from build123d import *

# Parameters (mm, degrees)
SKETCH1_R           = 2
BOSS_EXTRUDE1_DEPTH = 3.5
BOSS_EXTRUDE3_START = -1
BOSS_EXTRUDE3_DEPTH = 2
FILLET1_R           = 1


with BuildPart() as part:
    # Sketch1 → Boss-Extrude1 (new body)
    with BuildSketch(Plane.XY):
        with BuildLine():
            Line((-63.221147144, 4.5), (-2.221147144, 4.5))
            ThreePointArc((-2.221147144, 4.5), (1.924633844, -3.295084972), (-6.856271198, -2.375))
            ThreePointArc((-6.856271198, -2.375), (-7.960294648, -1.012531407), (-9.637345631, -0.5))
            Line((-9.637345631, -0.5), (-55.804948657, -0.5))
            ThreePointArc((-55.804948657, -0.5), (-57.48199964, -1.012531407), (-58.586023089, -2.375))
            ThreePointArc((-58.586023089, -2.375), (-67.366928132, -3.295084972), (-63.221147144, 4.5))
        make_face()
        with Locations((-63.221147144, -0.5)):
            Circle(SKETCH1_R, mode=Mode.SUBTRACT)
        with Locations((-2.221147144, -0.5)):
            Circle(SKETCH1_R, mode=Mode.SUBTRACT)
    extrude(amount=BOSS_EXTRUDE1_DEPTH)

    # Sketch3 → Boss-Extrude3 (add)
    with BuildSketch(Plane.XY.offset(3.5).offset(BOSS_EXTRUDE3_START)):
        with BuildLine():
            Line((-21.127237453, -1.361660316), (-19.026013205, -1.361660316))
            ThreePointArc((-19.026013205, -1.361660316), (-15.270540556, -0.058260327), (-19.221147144, -0.5))
            Line((-19.221147144, -0.5), (-21.221147144, -0.5))
            ThreePointArc((-21.221147144, -0.5), (-13.244693873, -0.066618664), (-21.127237453, -1.361660316))
        make_face()
    extrude(amount=-BOSS_EXTRUDE3_DEPTH)

    # Fillet1
    fillet1_edges = [part.edges().sort_by_distance(p)[0] for p in [
        (-13.221147144, -0.5, 1.5),
    ]]
    fillet(fillet1_edges, radius=FILLET1_R)


solid = part.part
Design review of the part built by this model. Coordinates are the model's own, in mm. A direction names the side the tool comes from. Coordinates: 2 decimals unless noted, no trailing zeros. Order: outer loops, then holes, each group sorted by start corner. A loop starts at its lowest first (then second) coordinate and runs counter-clockwise, first axis right, second up.
Item 1: Take a section at D-D, the plane y = 3.5. Write out the cut boundary in (x, z).
Item 2: The part is to be moulded in two halves that separate along X. For faces 5 (the flat face through (-32, 1, 0)), 6 (the flat face through (-17, -3, 0.5)), 7 (the cylindrical face through (-7.94, -1.027, 1.726)), say which applies: pulls with the +X half, pulls with the -X half, needs draft (parallel to the pull), parting line crosses it, or undercut.
Item 3: Take a section at B-B, the plane x = -3. Write out the cut boundary in (y, z), then the cut area to 3 significant figures.
Item 4: Take a section at A-A, the plane z = 1.1. Write out the cut boundary in (x, y) (3 decimals).
Item 5: For faces 1 (the flat face through (-17, -3, 2.5)), 2 (the flat face through (-33, 4.5, 2)), 3 (the cylindrical face through (-57.46, -1, 1.73)), 4 (the flat face through (-20, -1.362, 2)), list the 3-axis set-ups (+Z, -Z, +X, -X, +Y, -Y) from which the entire face can be reached by the end or side of a thin tool; tool diameter is ignored.
Item 6: For pin 1 Ø3 at (x, y) = (-2.22, -0.5) entering from +Z; pin 2 Ø3 at (x, y) = (-14.5, -2.5) entering from -Z; pin 3 Ø2 at (x, y) = (-16.5, -2) entering from +Z; pin 4 Ø4.5 at (x, y) = (-63.22, -0.5) entering from -Z, all flat-tipped, find the tip position at first contact; note any pin that passes through.
Item 7: Take a section at C-C, the plane x = -52.5. Write out the cut boundary in (y, z), then the cut area to 3 significant figures.
Item 8: For line 1 (Y direction, x = -17, z = 2.1); line 2 (X direction, y = 1.25, z = 0.3); line 3 (Y direction, x = -14, z = 3), list the stretches that pass through material, from the lowest coordinate up.
The answers:
1. outline: (-66.22, 0) - (0.78, 0) - (0.78, 3.5) - (-66.22, 3.5) - close
2. face 5: needs draft
2. face 6: undercut
2. face 7: undercut
3. outline: (-5.44, 0) - (-2.34, 0) - (-2.34, 3.5) - (-5.44, 3.5) - close; (1.34, 0) - (4.5, 0) - (4.5, 3.5) - (1.34, 3.5) - close
3. area: 21.9 mm2
4. outline: (-63.221, 4.5) arc R5 ccw (long way) to (-58.586, -2.375) arc R3 cw to (-55.805, -0.5) - (-15.221, -0.5) arc R2 cw to (-19.026, -1.362) - (-21.127, -1.362) arc R4 ccw to (-13.302, -1.3) arc R1 cw to (-12.322, -0.5) - (-9.637, -0.5) arc R3 cw to (-6.856, -2.375) arc R5 ccw (long way) to (-2.221, 4.5) - close; hole circle Ø4 at (-63.221, -0.5); hole circle Ø4 at (-2.221, -0.5)
5. face 1: +Z, -Y
5. face 2: +Z, -Z, +X, -X, +Y
5. face 3: +Z, -Z, -Y
5. face 4: +Z, -Z
6. pin 1: passes through
6. pin 2: stops at z = 0.5
6. pin 3: stops at z = 2.5
6. pin 4: stops at z = 0
7. outline: (-0.5, 0) - (4.5, 0) - (4.5, 3.5) - (-0.5, 3.5) - close
7. area: 17.5 mm2
8. line 1: y = -4.49 to -2.49, -0.5 to 4.5
8. line 2: x = -67.9 to -64.19, -62.25 to -3.19, -1.25 to 2.46
8. line 3: y = -0.5 to 4.5
